```python
from build123d import *

# Parameters (mm, degrees)
CUT_EXTRUDE_1_DEPTH = 3
FILLET_1_R          = 0.3
CHAMFER_1_SIZE      = 1


with BuildPart() as part:
    # Эскиз1 → Повернуть1 (revolve)
    with BuildSketch(Plane.XY):
        with BuildLine():
            Line((0, 0), (0, 5.5))
            ThreePointArc((0, 5.5), (2.128291755, 6.615124735), (4.5, 7))
            Line((4.5, 7), (5, 7))
            Line((5, 7), (5, 4))
            Line((5, 4), (35, 4))
            Line((35, 4), (35, 0))
            Line((35, 0), (0, 0))
        make_face()
    revolve(axis=Axis((35, 0, 0), (-1, 0, 0)))

    # Эскиз2 → Вырез-Вытянуть1 (cut)
    with BuildSketch(Plane.ZY):
        Polygon((1.732050808, 3), (-1.732050808, 3), (-3.464101615, 0), (-1.732050808, -3), (1.732050808, -3), (3.464101615, 0), align=None)
    extrude(amount=-CUT_EXTRUDE_1_DEPTH, mode=Mode.SUBTRACT)

    # Скругление1
    fillet_1_edges = [part.edges().sort_by_distance(p)[0] for p in [
        (5, -4, 0),
        (5, -7, 0),
    ]]
    fillet(fillet_1_edges, radius=FILLET_1_R)

    # Фаска1
    chamfer_1_edges = [part.edges().sort_by_distance(p)[0] for p in [
        (35, -4, 0),
    ]]
    chamfer(chamfer_1_edges, length=CHAMFER_1_SIZE)


solid = part.part
```
The listing builds one solid part. Answer for the finished solid, in the listing's coordinates (mm). A direction names the side the tool comes from. Coordinates: 2 decimals unless noted, no trailing zeros. Write each loop counter-clockwise with the first axis right and the second up, starting at its lowest first coordinate (ties: lowest second). Pieces come first, ordered by that corner, then holes. Notation, with made-up numbers: (46, 5.5) - (73, 5.5) arc R23 cw to (73, 34.5) - close; hole circle Ø2 at (12, 67). An arc over 180 degrees is marked (long way). Return JSON: item names as keys, results as strings. Group by question number.
Q1. For a pull along Z with two mould halves and no side action, classify faces 1 (the flat face through (5, 1.4, 4.4)), 2 (the flat face through (1.5, 1.5, 2.6)), 3 (the cylindrical face through (19.851, -0.867, 3.905)) as +Z half, -Z half, draft (parallel to the pull), parting line (faces both ways), or undercut.
Q2. Find the intervals of material crossed by line 1 along X through (y, z) = (2.5, -0.5); line 2 along X through (y, z) = (-4, -1.5); line 3 along Z through (x, y) = (21.5, -1), in increasing order. Write a range as [from, to].
Q3. Flat-ended cylindrical pins translate along their axes: pin 1 Ø5 at (x, y) = (9.5, -1.5) entering from +Z; pin 2 Ø1.5 at (x, z) = (22, 1.5) entering from -Y; pin 3 Ø4 at (x, z) = (18.5, -0.5) entering from +Y; pin 4 Ø4 at (y, z) = (-3, -3) entering from -X. Find the tip coordinate at first contact, or state that the pin passes through.
Q4. Which of the six approach directions +Z, -Z, +X, -X, +Y, -Y give full straight-line access (tool end or side, diameter ignored) to faces 4 (the flat face through (3, 0, 0)), 5 (the flat face through (0, -2.4, 2.4))?
Q5. The part is cut by section A-A on x = 11. Write down the section's boundary in (y, z).
Evaluation:
{
 "1": {"face 1": "draft", "face 2": "undercut", "face 3": "parting line"},
 "2": {"line 1": "x = [3, 35]", "line 2": "x = [0, 5]", "line 3": "z = [-3.87, 3.87]"},
 "3": {"pin 1": "stops at z = 4", "pin 2": "stops at y = -3.93", "pin 3": "stops at y = 4", "pin 4": "stops at x = 0"},
 "4": {"face 4": "-X", "face 5": "+Z, -Z, -X, +Y, -Y"},
 "5": {"outline": "circle Ø8 at (0, 0)"}
}
